from build123d import *

# Parameters (mm, degrees)
SKETCH1_W           = 70
SKETCH1_H           = 70
SKETCH1_R           = 3
SKETCH1_R_2         = 3.25
BOSS_EXTRUDE1_DEPTH = 3.1
SKETCH2_W           = 3.1
SKETCH2_H           = 35
BOSS_EXTRUDE2_DEPTH = 3.1
CUT_EXTRUDE1_DEPTH  = 4.1


with BuildPart() as part:
    # Sketch1 → Boss-Extrude1 (new body)
    with BuildSketch(Plane.XY):
        Rectangle(SKETCH1_W, SKETCH1_H)
        with Locations((-29.185832393, 29.185832393)):
            Circle(SKETCH1_R, mode=Mode.SUBTRACT)
        with Locations((29.185832393, 29.185832393)):
            Circle(SKETCH1_R, mode=Mode.SUBTRACT)
        with Locations((29.185832393, -29.185832393)):
            Circle(SKETCH1_R, mode=Mode.SUBTRACT)
        with Locations((-29.185832393, -29.185832393)):
            Circle(SKETCH1_R, mode=Mode.SUBTRACT)
        with Locations((15, 0)):
            Circle(SKETCH1_R_2, mode=Mode.SUBTRACT)
        with Locations((-15, 0)):
            Circle(SKETCH1_R_2, mode=Mode.SUBTRACT)
    extrude(amount=BOSS_EXTRUDE1_DEPTH)

    # Sketch2 → Boss-Extrude2 (add, through all)
    with BuildSketch(Plane.XY.offset(3.1)):
        with Locations((36.55, -17.5)):
            Rectangle(SKETCH2_W, SKETCH2_H)
        with Locations((-36.55, -17.5)):
            Rectangle(SKETCH2_W, SKETCH2_H)
    extrude(amount=-BOSS_EXTRUDE2_DEPTH)

    # Sketch3 → Cut-Extrude1 (cut, through all)
    with BuildSketch(Plane.XY.offset(3.1)):
        with BuildLine():
            Line((-15.911823751, 19.447357657), (-0.001921175, 3.537455081))
            Line((-0.001921175, 3.537455081), (15.907981402, 19.447357657))
            ThreePointArc((15.907981402, 19.447357657), (19.443515308, 19.447357657), (19.443515308, 15.911823751))
            Line((19.443515308, 15.911823751), (3.533612731, 0.001921175))
            Line((3.533612731, 0.001921175), (19.443515308, -15.907981402))
            ThreePointArc((19.443515308, -15.907981402), (19.443515308, -19.443515308), (15.907981402, -19.443515308))
            Line((15.907981402, -19.443515308), (-0.001921175, -3.533612731))
            Line((-0.001921175, -3.533612731), (-15.911823751, -19.443515308))
            ThreePointArc((-15.911823751, -19.443515308), (-19.447357657, -19.443515308), (-19.447357657, -15.907981402))
            Line((-19.447357657, -15.907981402), (-3.537455081, 0.001921175))
            Line((-3.537455081, 0.001921175), (-19.447357657, 15.911823751))
            ThreePointArc((-19.447357657, 15.911823751), (-19.447357657, 19.447357657), (-15.911823751, 19.447357657))
        make_face()
    extrude(amount=-CUT_EXTRUDE1_DEPTH, mode=Mode.SUBTRACT)


solid = part.part
Can you work these out from the model? Positions are in its coordinate system, mm. A direction names the side the tool comes from. Give positions to 0.01 mm unless a question says otherwise; leave off trailing zeros. Order: outer loops, then holes, each group sorted by start corner. A loop starts at its lowest first (then second) coordinate and runs counter-clockwise, first axis right, second up. Notation, with made-up numbers: M -27.5,5.25 L -14.5,5.25 A7 cw -14.5,9.25 Z; hole C 73.25,-39.5 d8. An arc over 180 degrees is marked long. One line per question, with ' | ' between items.
Item 1: Suppose I cut it at C-C, the plane x = 6. Write out the boundary of the cut face in (y, z), then the cut area to 3 significant figures.
Answer block:
outline: M -35,0 L -9.54,0 L -9.54,3.1 L -35,3.1 Z; M -2.46,0 L 2.47,0 L 2.47,3.1 L -2.46,3.1 Z; M 9.54,0 L 35,0 L 35,3.1 L 9.54,3.1 Z | area: 173 mm2
Item 2: For faces 1 (the face through (-35, 17, 2)), 2 (the face through (-11.6, -8.06, 1.57)), 3 (the face through (37, 0, 2)), which set-ups out of +Z, -Z, +X, -X, +Y, -Y let a thin tool reach every point of the face, with its end or its side?
Answer block:
face 1: +Z, -Z, -X, +Y | face 2: +Z, -Z | face 3: +Z, -Z, +X, +Y
Item 3: I'm going to push a flat-ended pin straight in: pin 1 Ø1.6 at (y, z) = (15, 1.5) entering from +X. Where does the tip first touch, or does it pass through?
Answer block:
pin 1: stops at x = 35
Item 4: Suppose I cut it at A-A, the plane x = -15. Write out the boundary of the cut face in (y, z).
Answer block:
outline: M -35,0 L -18.53,0 L -18.53,3.1 L -35,3.1 Z; M -11.46,0 L -3.25,0 L -3.25,3.1 L -11.46,3.1 Z; M 3.25,0 L 11.46,0 L 11.46,3.1 L 3.25,3.1 Z; M 18.54,0 L 35,0 L 35,3.1 L 18.54,3.1 Z
Item 5: We'd pull the mould along Y, two halves only. Please class faces 4 (the face through (0, 35, 2)), 5 (the face through (-1, -35, 2)), 6 (the face through (-38.1, -18, 2)), 7 (the face through (11.6, 8.07, 1.57)): released by +Y, released by -Y, zero draft, split by the parting line, or undercut.
Answer block:
face 4: released by +Y | face 5: released by -Y | face 6: zero draft | face 7: undercut
Item 6: Suppose I cut it at D-D, the plane z = 0.55. Write out the boundary of the cut face in (x, y).
Answer block:
outline: M -38.1,-35 L 38.1,-35 L 38.1,0 L 35,0 L 35,35 L -35,35 L -35,0 L -38.1,0 Z; hole C -29.19,-29.19 d6; hole C -29.19,29.19 d6; hole M -19.45,-15.91 A2.5 ccw -15.91,-19.44 L 0,-3.53 L 15.91,-19.44 A2.5 ccw 19.44,-15.91 L 3.53,0 L 19.44,15.91 A2.5 ccw 15.91,19.45 L 0,3.54 L -15.91,19.45 A2.5 ccw -19.45,15.91 L -3.54,0 Z; hole C -15,0 d6.5; hole C 15,0 d6.5; hole C 29.19,-29.19 d6; hole C 29.19,29.19 d6
Item 7: Please list where these lines run through material, in increasing order: L1, parallel to Y at x = 29.5, z = 1.7; L2, parallel to X at y = -7, z = 0.8; L3, parallel to Y at x = -16.5, z = 2.6.
Answer block:
L1: y = -35 to -32.17, -26.2 to 26.2, 32.17 to 35 | L2: x = -38.1 to -10.54, -3.47 to 3.46, 10.54 to 38.1 | L3: y = -35 to -19.88, -12.96 to -2.88, 2.88 to 12.96, 19.88 to 35
Item 8: Suppose I cut it at B-B, the plane y = 30.5. Write out the boundary of the cut face in (x, z).
Answer block:
outline: M -35,0 L -31.88,0 L -31.88,3.1 L -35,3.1 Z; M -26.49,0 L 26.49,0 L 26.49,3.1 L -26.49,3.1 Z; M 31.88,0 L 35,0 L 35,3.1 L 31.88,3.1 Z
